Design review of the part built by this model. Coordinates are the model's own, in mm. A direction names the side the tool comes from. Give positions to 0.01 mm unless a question says otherwise; leave off trailing zeros. Write each loop counter-clockwise with the first axis right and the second up, starting at its lowest first coordinate (ties: lowest second). Pieces come first, ordered by that corner, then holes. Notation, with made-up numbers: (73, -5) -> (94, -5) arc R17 cw to (94, 9) -> close; hole circle Ø11 at (-15.5, 23). An arc over 180 degrees is marked (long way). Write each question's results on one line, items separated by ' | '. Start each with the question number.
(1) For faces 4 (the face through (43, -78, -29)), 5 (the face through (43, -64, -29)), 6 (the face through (-72, -45, -37)), list the 3-axis set-ups (+Z, -Z, +X, -X, +Y, -Y) from which the entire face can be reached by the end or side of a thin tool; tool diameter is ignored.
(2) Take a section at A-A (y = -22). State the section outline as (x, z) points.
(3) Clearance check with flat-ended pins moving along their axes: pin 1 (2.5 mm diameter, centred on y = -78, z = 8, fed in from -X); pin 2 (5.5 mm diameter, centred on x = 45.5, y = -46.5, fed in from +Z); pin 3 (10 mm diameter, centred on x = 21, z = 9, fed in from -Y). State where each tip first meets the part, or that it passes through.
(4) Mouldability with a two-part tool opening along X and no side actions: class faces 1 (the face through (-80, -32, -30)), 2 (the face through (6, -45, -1)), 3 (the face through (-78, -45, -29)) as released by +X, released by -X, zero draft, split by the parting line, or undercut.
(5) Take a section at D-D (x = 24). State the section outline as (y, z) points.
(6) To check wall thickness, follow probe 1 along Y at (x, z) = (39, 13); probe 2 along X at (y, z) = (-59, -9); probe 3 along X at (y, z) = (-53.5, -34). State the ranges of each line that lie inside material, in increasing order.
(7) Take a section at C-C (z = -33). State the section outline as (x, y) points, plus the area to 3 significant figures.
(8) Take a section at B-B (z = -20). State the section outline as (x, y) points.
from build123d import *

# Parameters (mm, degrees)
F0_W      = 160
F0_H      = 82
F1_DEPTH  = 10
F2_W      = 12
F2_H      = 12
F3_DEPTH  = 70
F4_W      = 74
F4_H      = 12
F5_DEPTH  = 70
F6_W      = 5
F6_H      = 70
F7_DEPTH  = 70
F8_W      = 64
F8_H      = 5
F9_DEPTH  = 80
F10_W     = 8
F10_H     = 8
F11_DEPTH = 70
F12_W     = 8
F12_H     = 8
F13_DEPTH = 70
F14_SIZE  = 1
F15_SIZE  = 1
F16_SIZE  = 1
F17_SIZE  = 1
F18_SIZE  = 1
F19_SIZE  = 1
F20_SIZE  = 1
F21_SIZE  = 1
F22_SIZE  = 1
F23_SIZE  = 1
F24_SIZE  = 1
F25_SIZE  = 1
F26_SIZE  = 1
F27_SIZE  = 1


with BuildPart() as f1:
    # F0 (on Front) → F1 (new body)
    with BuildSketch(Plane.XZ):
        Rectangle(F0_W, F0_H)
    extrude(amount=F1_DEPTH)

    # F2 (on face) → F3 (join)
    with BuildSketch(Plane.XZ.offset(10)):
        with Locations((-74, 35)):
            Rectangle(F2_W, F2_H)
        with Locations((-74, -35)):
            Rectangle(F2_W, F2_H)
    extrude(amount=F3_DEPTH)

    # F4 (on face) → F5 (join)
    with BuildSketch(Plane.XZ.offset(10)):
        with Locations((43, -35)):
            Rectangle(F4_W, F4_H)
    extrude(amount=F5_DEPTH)

    # F6 (on face) → F7 (join)
    with BuildSketch(Plane.XZ.offset(10)):
        with Locations((8.5, 6)):
            Rectangle(F6_W, F6_H)
        with Locations((77.5, 6)):
            Rectangle(F6_W, F6_H)
    extrude(amount=F7_DEPTH)

    # F8 (on face) → F9 (join)
    with BuildSketch(Plane.XY.offset(41)):
        with Locations((43, -30.5)):
            Rectangle(F8_W, F8_H)
        with Locations((43, -53.5)):
            Rectangle(F8_W, F8_H)
        with Locations((43, -74.3680498004)):
            Rectangle(F8_W, F8_H)
    extrude(amount=-F9_DEPTH)

    # F10 (on face) → F11 (cut)
    with BuildSketch(Plane.XZ.offset(80)):
        with Locations((-72, 33)):
            Rectangle(F10_W, F10_H)
    extrude(amount=-F11_DEPTH, mode=Mode.SUBTRACT)

    # F12 (on face) → F13 (cut)
    with BuildSketch(Plane.XZ.offset(80)):
        with Locations((-72, -33)):
            Rectangle(F12_W, F12_H)
    extrude(amount=-F13_DEPTH, mode=Mode.SUBTRACT)

    # F14
    f14_edges = [f1.edges().sort_by_distance(p)[0] for p in [
        (-80, 0, 0),
    ]]
    chamfer(f14_edges, length=F14_SIZE)

    # F15
    f15_edges = [f1.edges().sort_by_distance(p)[0] for p in [
        (0.5, 0, 41),
    ]]
    chamfer(f15_edges, length=F15_SIZE)

    # F16
    f16_edges = [f1.edges().sort_by_distance(p)[0] for p in [
        (80, 0, -0.5),
    ]]
    chamfer(f16_edges, length=F16_SIZE)

    # F17
    f17_edges = [f1.edges().sort_by_distance(p)[0] for p in [
        (0, 0, -41),
    ]]
    chamfer(f17_edges, length=F17_SIZE)

    # F18
    f18_edges = [f1.edges().sort_by_distance(p)[0] for p in [
        (-80, -40.5, 41),
    ]]
    chamfer(f18_edges, length=F18_SIZE)

    # F19
    f19_edges = [f1.edges().sort_by_distance(p)[0] for p in [
        (80, -40.5, 41),
    ]]
    chamfer(f19_edges, length=F19_SIZE)

    # F20
    f20_edges = [f1.edges().sort_by_distance(p)[0] for p in [
        (-80, -40.5, -41),
    ]]
    chamfer(f20_edges, length=F20_SIZE)

    # F21
    f21_edges = [f1.edges().sort_by_distance(p)[0] for p in [
        (80, -40.5, -41),
    ]]
    chamfer(f21_edges, length=F21_SIZE)

    # F22
    f22_edges = [f1.edges().sort_by_distance(p)[0] for p in [
        (6, -45, -41),
    ]]
    chamfer(f22_edges, length=F22_SIZE)

    # F23
    f23_edges = [f1.edges().sort_by_distance(p)[0] for p in [
        (-31, -10, -41),
    ]]
    chamfer(f23_edges, length=F23_SIZE)

    # F24
    f24_edges = [f1.edges().sort_by_distance(p)[0] for p in [
        (-68, -45, -41),
    ]]
    chamfer(f24_edges, length=F24_SIZE)

    # F25
    f25_edges = [f1.edges().sort_by_distance(p)[0] for p in [
        (-31, -10, 41),
    ]]
    chamfer(f25_edges, length=F25_SIZE)

    # F26
    f26_edges = [f1.edges().sort_by_distance(p)[0] for p in [
        (-68, -45, 41),
    ]]
    chamfer(f26_edges, length=F26_SIZE)

    # F27
    f27_edges = [f1.edges().sort_by_distance(p)[0] for p in [
        (6, -45, 41),
    ]]
    chamfer(f27_edges, length=F27_SIZE)


solid = f1.part
Report:
1) face 4: +Z, -Y | face 5: +Z | face 6: -Y
2) outline: (-80, -40) -> (-79, -41) -> (-69, -41) -> (-68, -40) -> (-68, -37) -> (-76, -37) -> (-76, -29) -> (-80, -29) -> close; (-80, 29) -> (-76, 29) -> (-76, 37) -> (-68, 37) -> (-68, 40) -> (-69, 41) -> (-79, 41) -> (-80, 40) -> close; (6, -40) -> (7, -41) -> (79, -41) -> (80, -40) -> (80, 40) -> (79, 41) -> (75, 41) -> (75, -29) -> (11, -29) -> (11, 41) -> (7, 41) -> (6, 40) -> close
3) pin 1: x = 6 | pin 2: z = -29 | pin 3: y = -76.87
4) face 1: released by -X | face 2: undercut | face 3: zero draft
5) outline: (-80, -41) -> (-1, -41) -> (0, -40) -> (0, 40) -> (-1, 41) -> (-10, 41) -> (-10, -29) -> (-28, -29) -> (-28, 41) -> (-33, 41) -> (-33, -29) -> (-51, -29) -> (-51, 41) -> (-56, 41) -> (-56, -29) -> (-71.87, -29) -> (-71.87, 41) -> (-76.87, 41) -> (-76.87, -29) -> (-80, -29) -> close
6) probe 1: -76.87 to -71.87, -56 to -51, -33 to -28, -10 to 0 | probe 2: 6 to 11, 75 to 80 | probe 3: -80 to -76, 6 to 80
7) outline: (-80, -80) -> (-76, -80) -> (-76, -10) -> (6, -10) -> (6, -80) -> (80, -80) -> (80, -1) -> (79, 0) -> (-79, 0) -> (-80, -1) -> close | area: 7,060 mm2
8) outline: (-80, -10) -> (6, -10) -> (6, -80) -> (11, -80) -> (11, -76.87) -> (75, -76.87) -> (75, -80) -> (80, -80) -> (80, -1) -> (79, 0) -> (-79, 0) -> (-80, -1) -> close; hole (11, -71.87) -> (75, -71.87) -> (75, -56) -> (11, -56) -> close; hole (11, -51) -> (75, -51) -> (75, -33) -> (11, -33) -> close; hole (11, -28) -> (75, -28) -> (75, -10) -> (11, -10) -> close
